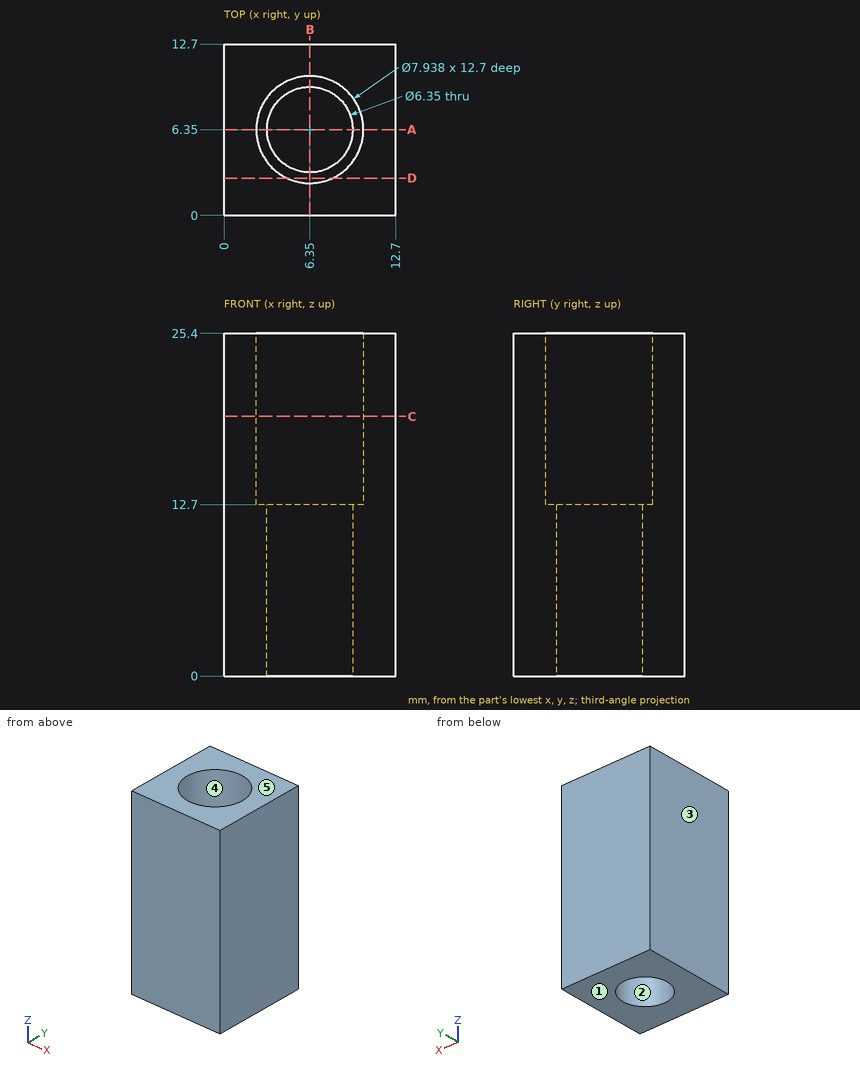
Verification items for this drawing (mm, ordinates from the low corner). A direction names the side the tool comes from. Coordinates: 2 decimals unless noted, no trailing zeros. Order: outer loops, then holes, each group sorted by start corner. A loop starts at its lowest first (then second) coordinate and runs counter-clockwise, first axis right, second up. Notation, with made-up numbers: (79.5, -13.5) - (109.5, -13.5) arc R17 cw to (109.5, 17.5) - close; hole circle Ø9 at (53.25, -11). An arc over 180 degrees is marked (long way). Answer in a Markdown table with one row per item. Add a question column.
1. Section check C-C (z = 19.25). Enter the section's corners in (x, y).
2. Draft check along X on the marked faces 1, 2 and 3. Enter one of: +X half, -X half, draft (parallel to the pull), parting line (faces both ways), or undercut.
3. Section check A-A (y = 6.35). Enter the section's corners in (x, z) (1 decimal), plus the area to 3 significant figures.
4. Material ranges on L1, parallel to Y at x = 6.35, z = 20.25; L2, parallel to X at y = 6.5, z = 19 (1 decimal); L3, parallel to Y at x = 6.35, z = 6.75 (1 decimal), recorded low to high. Write a range as [from, to].
5. Section check D-D (y = 2.75). Enter the section's corners in (x, z), plus the area to 3 significant figures.
6. Gauge pin test, flat end, axial feed: pin 1 Ø6.5 at (x, y) = (6.35, 6.35) entering from -Z. Record the tip position at first contact, or that the pin passes through.
7. Access from +Z, -Z, +X, -X, +Y, -Y to the whole of each face (thin tool, end or side, straight path). Record for the marked faces 4 and 5.
Data:
| question | item | result |
|---|---|---|
| 1 | outline | (0, 0) - (12.7, 0) - (12.7, 12.7) - (0, 12.7) - close; hole circle Ø7.94 at (6.35, 6.35) |
| 2 | face 1 | draft |
| 2 | face 2 | undercut |
| 2 | face 3 | -X half |
| 3 | outline | (0, 0) - (3.2, 0) - (3.2, 12.7) - (2.4, 12.7) - (2.4, 25.4) - (0, 25.4) - close; (9.5, 0) - (12.7, 0) - (12.7, 25.4) - (10.3, 25.4) - (10.3, 12.7) - (9.5, 12.7) - close |
| 3 | area | 141 mm² |
| 4 | L1 | y = [0, 2.38], [10.32, 12.7] |
| 4 | L2 | x = [0, 2.4], [10.3, 12.7] |
| 4 | L3 | y = [0, 3.2], [9.5, 12.7] |
| 5 | outline | (0, 0) - (12.7, 0) - (12.7, 25.4) - (8.02, 25.4) - (8.02, 12.7) - (4.68, 12.7) - (4.68, 25.4) - (0, 25.4) - close |
| 5 | area | 280 mm² |
| 6 | pin 1 | stops at z = 0 |
| 7 | face 4 | +Z |
| 7 | face 5 | +Z, +X, -X, +Y, -Y |
